Read the model definition and answer for the solid it produces. Units are mm, in the model's axes. A direction names the side the tool comes from. Give positions to 0.01 mm unless a question says otherwise; leave off trailing zeros. Order: outer loops, then holes, each group sorted by start corner. A loop starts at its lowest first (then second) coordinate and runs counter-clockwise, first axis right, second up. Notation, with made-up numbers: (-13.5, 85) -> (16.5, 85) arc R21 cw to (16.5, 123) -> close; hole circle Ø3 at (84, 42). An arc over 180 degrees is marked (long way). Use one line per item in the form item = value.
```python
from build123d import *

# Parameters (mm, degrees)
BOSS_EXTRUDE1_DEPTH   = 14
BOSS_EXTRUDE1_2_DEPTH = 14
BOSS_EXTRUDE2_DEPTH   = 14
SKETCH3_R             = 0.6
CUT_EXTRUDE1_DEPTH    = 15


with BuildPart() as part:
    # Sketch2 → Boss-Extrude1 (new body)
    with BuildSketch(Plane(origin=(0, 0, 0), x_dir=(1, 0, 0), z_dir=(0, 1, 0))):
        Polygon((7.717934448, -19.134647491), (-1.99762589, -9.419087153), (-1.562483255, -8.440016225), (7.717934448, -17.720433929), align=None)
    extrude(amount=BOSS_EXTRUDE1_DEPTH)



with BuildPart() as body_2:
    # Sketch2 → Boss-Extrude1 2 (new body)
    with BuildSketch(Plane(origin=(0, 0, 0), x_dir=(1, 0, 0), z_dir=(0, 1, 0))):
        Polygon((7.717934448, -5.761075504), (2.117319337, -0.160460393), (2.552461971, 0.818610535), (7.717934448, -4.346861942), align=None)
    extrude(amount=BOSS_EXTRUDE1_2_DEPTH)


with BuildPart() as part_1:
    add(part.part)

    add(body_2.part)  # Boss-Extrude2 merges body 2
    # Sketch1 → Boss-Extrude2 (add)
    with BuildSketch(Plane(origin=(0, 0, 0), x_dir=(1, 0, 0), z_dir=(0, 1, 0))):
        Polygon((-10.282065552, -23.134647491), (8.717934448, 19.615352509), (9.717934448, 19.615352509), (9.717934448, -23.134647491), (9.717934448, -26.134647491), (-10.282065552, -26.134647491), align=None)
        Polygon((7.717934448, -21.134647491), (7.717934448, 12.440923608), (-7.204541596, -21.134647491), align=None, mode=Mode.SUBTRACT)
    extrude(amount=BOSS_EXTRUDE2_DEPTH)

    # Sketch3 → Cut-Extrude1 (cut, through all)
    with BuildSketch(Plane(origin=(0, 14, 0), x_dir=(1, 0, 0), z_dir=(0, 1, 0))):
        with Locations((4.717934448, -24.134647491)):
            Circle(SKETCH3_R)
        with Locations((-5.282065552, -24.134647491)):
            Circle(SKETCH3_R)
    extrude(amount=-CUT_EXTRUDE1_DEPTH, mode=Mode.SUBTRACT)


solid = part_1.part
```
Item 1: The part is cut by section B-B on z = -4. Give the vertices of the cut face in (x, y), and give its area (3 significant figures).
Checks:
outline = (1.78, 0) -> (3.97, 0) -> (3.97, 14) -> (1.78, 14) -> close; (7.72, 0) -> (9.72, 0) -> (9.72, 14) -> (7.72, 14) -> close
area = 58.6 mm²
Item 2: Determine the mould class of faces 3 (the flat face through (-10.282, 7, 25)), 4 (the flat face through (-0.915, 6.902, 2.059)), 5 (the flat face through (7.718, 7, 12)) for opening direction Z: +Z half, -Z half, draft (parallel to the pull), parting line (faces both ways), or undercut.
Checks:
face_3 = draft
face_4 = -Z half
face_5 = undercut
Item 3: The part is cut by section A-A on z = 14. Give the vertices of the cut face in (x, y), and give its area (3 significant figures).
Checks:
outline = (-6.22, 0) -> (-4.03, 0) -> (-4.03, 14) -> (-6.22, 14) -> close; (2.58, 0) -> (4, 0) -> (4, 14) -> (2.58, 14) -> close; (7.72, 0) -> (9.72, 0) -> (9.72, 14) -> (7.72, 14) -> close
area = 78.4 mm²
Item 4: Which of the six approach directions +Z, -Z, +X, -X, +Y, -Y give full straight-line access (tool end or side, diameter ignored) to faces 1 (the flat face through (9, 7, -19.615)), 2 (the flat face through (7.718, 7, -4))?
Checks:
face_1 = -Z, +X, -X, +Y, -Y
face_2 = +Y, -Y
Item 5: The part is cut by section C-C on x = -3.25. Give the vertices of the cut face in (y, z), and give its area (3 significant figures).
Checks:
outline = (0, 7.31) -> (14, 7.31) -> (14, 12.24) -> (0, 12.24) -> close; (0, 21.13) -> (14, 21.13) -> (14, 26.13) -> (0, 26.13) -> close
area = 139 mm²
Item 6: Straight lines are drawn through the part: L1, parallel to Z at x = -5.75, y = 7.5; L2, parallel to X at y = 8.5, z = 14; L3, parallel to Z at x = 7.5, y = 5.5 (1 decimal). For each, find the intervals that lie inside material, in ascending order. Write a range as from..to.
Checks:
L1 = 12.94..17.86, 21.13..23.76, 24.51..26.13
L2 = -6.22..-4.03, 2.58..4, 7.72..9.72
L3 = -16.9..-12, 4.1..5.5, 17.5..18.9, 21.1..26.1
Item 7: Given pin 1 Ø8 at (x, y) = (1, 8) entering from -Z; pin 2 Ø7 at (x, y) = (-3, 6) entering from -Z (3 decimals); pin 3 Ø2 at (y, z) = (6.5, 20.5) entering from -X, each flat-ended and moving along its own axis, determine where each tip first touches the part or whether it passes through.
Checks:
pin_1 = -11.25
pin_2 = -1.125
pin_3 = -9.56
Item 8: The part is cut by section D-D on x = 3. Give the vertices of the cut face in (y, z), and give its area (3 significant figures).
Checks:
outline = (0, -6.75) -> (14, -6.75) -> (14, -1.83) -> (0, -1.83) -> close; (0, -0.37) -> (14, -0.37) -> (14, 1.04) -> (0, 1.04) -> close; (0, 13) -> (14, 13) -> (14, 14.42) -> (0, 14.42) -> close; (0, 21.13) -> (14, 21.13) -> (14, 26.13) -> (0, 26.13) -> close
area = 179 mm²
